Geometry check sheet. Reference: the model listing, model coordinates, mm. Face numbers are marked on the shaded views. A direction names the side the tool comes from. Coordinates: 2 decimals unless noted, no trailing zeros. Write each loop counter-clockwise with the first axis right and the second up, starting at its lowest first coordinate (ties: lowest second). Pieces come first, ordered by that corner, then holes. Notation, with made-up numbers: M 3,51.25 L 16,51.25 A17 ccw 16,55.25 Z; hole C 67.5,35 d8. An arc over 180 degrees is marked long. Answer as a JSON object with one key per item and string values. Group by question number.
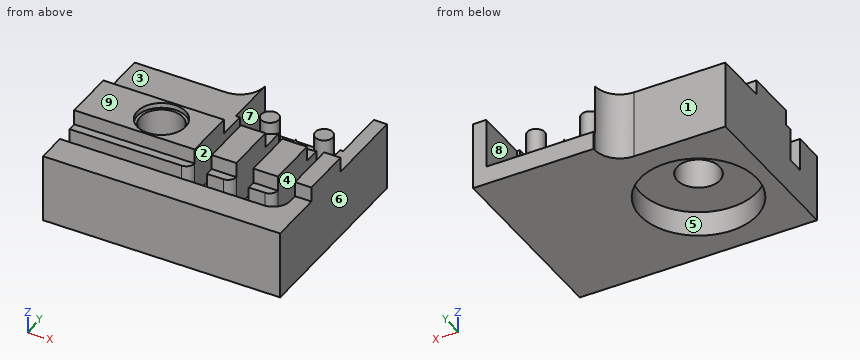
```python
from build123d import *

# Parameters (mm, degrees)
PAD004_DEPTH    = 8.2
SKETCH014_W     = 28.5
SKETCH014_H     = 6.2
PAD005_DEPTH    = 1.8
SKETCH015_R     = 2.9
POCKET004_DEPTH = 0.6
SKETCH016_W     = 2.05
SKETCH016_H     = 6.2
POCKET005_DEPTH = 1.8
SKETCH018_R     = 1.05
POCKET007_DEPTH = 6
POCKET006_DEPTH = 4
SKETCH019_R     = 2.55
POCKET008_DEPTH = 7.5
SKETCH020_R     = 7
POCKET_DEPTH    = 3


with BuildPart() as stage_1_railguide:
    # Sketch013 → Pad004 (new body)
    with BuildSketch(Plane.XY):
        with BuildLine():
            Line((0, 0), (28.5, 0))
            Line((28.5, 0), (28.5, 22.75))
            Line((28.5, 22.75), (14, 22.75))
            Line((14, 22.75), (14, 22.5))
            ThreePointArc((11, 19.5), (13.12132, 20.37868), (14, 22.5))
            Line((11, 19.5), (0, 19.5))
            Line((0, 19.5), (0, 0))
        make_face()
    extrude(amount=PAD004_DEPTH)

    # Sketch014 (on Face9 of Pad004) → Pad005 (join)
    with BuildSketch(Plane.XY.offset(8.2)):
        with Locations((14.25, 9.75)):
            Rectangle(SKETCH014_W, SKETCH014_H)
    extrude(amount=PAD005_DEPTH)

    # Sketch015 (on Face11 of Pad005) → Pocket004 (cut)
    with BuildSketch(Plane.XY.offset(10)):
        with Locations((8.735056, 9.75)):
            Circle(SKETCH015_R)
    extrude(amount=-POCKET004_DEPTH, mode=Mode.SUBTRACT)

    # Sketch016 (on Face10 of Pocket004) → Pocket005 (cut)
    with BuildSketch(Plane.XY.offset(10)):
        with Locations((15.5, 9.75)):
            Rectangle(SKETCH016_W, SKETCH016_H)
        Polygon((21.525, 12.85), (21.525, 6.65), (19.475, 6.65), (19.475, 12.85), (20.5, 12.85), align=None)
        with Locations((25.5, 9.75)):
            Rectangle(SKETCH016_W, SKETCH016_H)
    extrude(amount=-POCKET005_DEPTH, mode=Mode.SUBTRACT)


with BuildPart() as body:
    # Body006 base: copy of Stage#1(RailGuide)
    add(stage_1_railguide.part)

    # Sketch018 (on Face19 of Clone001) → Pocket007 (cut)
    with BuildSketch(Plane.XY.offset(8.2)):
        with BuildLine():
            Line((14, 22.75), (26.9, 22.75))
            Line((26.9, 22.75), (26.9, 16.25))
            Line((26.355184, 16.25), (26.9, 16.25))
            ThreePointArc((21.044816, 16.25), (23.7, 14.75), (26.355184, 16.25))
            Line((20.45, 16.25), (21.044816, 16.25))
            Line((19.855184, 16.25), (20.45, 16.25))
            ThreePointArc((14.544816, 16.25), (17.2, 14.75), (19.855184, 16.25))
            Line((14, 16.25), (14.544816, 16.25))
            Line((14, 16.25), (14, 22.75))
        make_face()
        with Locations((17.2, 17.85)):
            Circle(SKETCH018_R, mode=Mode.SUBTRACT)
        with Locations((23.7, 17.85)):
            Circle(SKETCH018_R, mode=Mode.SUBTRACT)
    extrude(amount=-POCKET007_DEPTH, mode=Mode.SUBTRACT)


with BuildPart() as body008:
    # Body005 base: copy of Stage#1(RailGuide)
    add(stage_1_railguide.part)

    # Sketch017 (on Face19 of Clone) → Pocket006 (cut)
    with BuildSketch(Plane.XY.offset(8.2)):
        with BuildLine():
            Line((0, 5.65), (13.475, 5.65))
            ThreePointArc((13.475, 5.65), (14.182107, 5.942893), (14.475, 6.65))
            Line((14.475, 6.65), (14.475, 16.75))
            Line((14.475, 16.75), (16.525, 16.75))
            Line((16.525, 16.75), (16.525, 5.65))
            Line((16.525, 5.65), (18.475, 5.65))
            ThreePointArc((18.475, 5.65), (19.182107, 5.942893), (19.475, 6.65))
            Line((19.475, 6.65), (19.475, 16.75))
            Line((19.475, 16.75), (21.525, 16.75))
            Line((21.525, 16.75), (21.525, 5.649972))
            Line((21.525, 5.649972), (23.475, 5.649972))
            ThreePointArc((23.475, 5.649972), (24.182107, 5.942865), (24.475, 6.649972))
            Line((24.475, 6.649972), (24.475, 16.75))
            Line((24.475, 16.75), (26.525, 16.75))
            Line((26.525, 16.75), (26.525, 5.65))
            ThreePointArc((24.475, 3.6), (25.924569, 4.200431), (26.525, 5.65))
            Line((24.475, 3.6), (0, 3.6))
            Line((0, 3.6), (0, 5.65))
        make_face()
    extrude(amount=-POCKET006_DEPTH, mode=Mode.SUBTRACT)

    # Sketch019 (on Face37 of Pocket006) → Pocket008 (cut)
    with BuildSketch(Plane.XY.offset(9.4)):
        with Locations((8.735056, 9.75)):
            Circle(SKETCH019_R)
    extrude(amount=-POCKET008_DEPTH, mode=Mode.SUBTRACT)

    # Sketch020 (on Face4 of Pocket008) → Pocket (cut)
    with BuildSketch(Plane(origin=(0, 0, 0), x_dir=(1, 0, 0), z_dir=(0, 0, -1))):
        with Locations((8.735056, -9.75)):
            Circle(SKETCH020_R)
    extrude(amount=-POCKET_DEPTH, mode=Mode.SUBTRACT)

    # Common: intersect Body
    add(body.part, mode=Mode.INTERSECT)


solid = body008.part
```
1) Set-up check for the marked faces 1, 2, 3, 4 and 5: record each of +Z, -Z, +X, -X, +Y, -Y from which the full face is reachable in a straight line by a thin tool's end or side.
2) Go/stop test with flat-tipped pins: pin 1 Ø6.5 at (x, y) = (8.74, 9.75) entering from -Z; pin 2 Ø1.1 at (x, y) = (23.5, 6) entering from +Z; pin 3 Ø0.5 at (x, z) = (18, 9.5) entering from -Y. Record where each tip stops, or that it passes through.
3) Material ranges on probe 1 along Y at (x, z) = (3.25, 7.75); probe 2 along Z at (x, y) = (3.75, 4); probe 3 along Z at (x, y) = (8.25, 17), recorded low to high. Write a range as [from, to].
4) Draft check along X on the marked faces 6, 7, 8 and 9. Enter one of: +X half, -X half, draft (parallel to the pull), parting line (faces both ways), or undercut.
5) Section check C-C (z = 1.75). Record the cut outline in (x, y), then the cut area to 3 significant figures.
6) Section check A-A (z = 3.5). Record the cut outline in (x, y), then the cut area to 3 significant figures.
7) Section check B-B (y = 9.75). Record the cut outline in (x, z) (3 decimals).
8) Section check D-D (y = 17.85). Record the cut outline in (x, z), then the cut area to 4 significant figures.
Entries:
{
 "1": {"face 1": "+Z, -Z, -X, +Y", "face 2": "+Z, +Y", "face 3": "+Z, +X, -X, +Y", "face 4": "+Z", "face 5": "-Z"},
 "2": {"pin 1": "z = 3", "pin 2": "z = 8.2", "pin 3": "y = 6.65"},
 "3": {"probe 1": "[0, 3.6], [5.65, 19.5]", "probe 2": "[0, 4.2]", "probe 3": "[0, 8.2]"},
 "4": {"face 6": "+X half", "face 7": "undercut", "face 8": "undercut", "face 9": "draft"},
 "5": {"outline": "M 0,0 L 28.5,0 L 28.5,22.75 L 14,22.75 L 14,22.5 A3 cw 11,19.5 L 0,19.5 Z; hole C 8.74,9.75 d14", "area": "451 mm^2"},
 "6": {"outline": "M 0,0 L 28.5,0 L 28.5,22.75 L 26.9,22.75 L 26.9,16.25 L 26.36,16.25 A3.1 cw 21.04,16.25 L 19.86,16.25 A3.1 cw 14.54,16.25 L 14,16.25 L 14,22.5 A3 cw 11,19.5 L 0,19.5 Z; C 17.2,17.85 d2.1; C 23.7,17.85 d2.1; hole C 8.74,9.75 d5.1", "area": "496 mm^2"},
 "7": {"outline": "M 0,0 L 1.735,0 L 1.735,3 L 6.185,3 L 6.185,9.4 L 5.835,9.4 L 5.835,10 L 0,10 Z; M 11.285,3 L 15.735,3 L 15.735,0 L 28.5,0 L 28.5,10 L 26.525,10 L 26.525,4.2 L 24.475,4.2 L 24.475,10 L 21.525,10 L 21.525,4.2 L 19.475,4.2 L 19.475,10 L 16.525,10 L 16.525,4.2 L 14.475,4.2 L 14.475,10 L 11.635,10 L 11.635,9.4 L 11.285,9.4 Z"},
 "8": {"outline": "M 0,0 L 28.5,0 L 28.5,8.2 L 26.9,8.2 L 26.9,2.2 L 24.75,2.2 L 24.75,8.2 L 22.65,8.2 L 22.65,2.2 L 18.25,2.2 L 18.25,8.2 L 16.15,8.2 L 16.15,2.2 L 14,2.2 L 14,8.2 L 0,8.2 Z", "area": "181.5 mm^2"}
}
